from build123d import *

# Parameters (mm, degrees)
SKETCH1_W                       = 39
SKETCH1_H                       = 155
BOSS_EXTRUDE1_DEPTH             = 2
BOSS_EXTRUDE2_DEPTH             = 38
SKETCH3_W                       = 2
SKETCH3_H                       = 2
BOSS_EXTRUDE3_DEPTH             = 38
SKETCH4_W                       = 2
SKETCH4_H                       = 2
BOSS_EXTRUDE4_DEPTH             = 151
SKETCH6_W                       = 35
SKETCH6_H                       = 2.2
CUT_EXTRUDE1_DEPTH              = 160.340045186
SKETCH7_W                       = 35
SKETCH7_H                       = 2.2
CUT_EXTRUDE2_DEPTH              = 89.490112442
SKETCH5_W                       = 31
SKETCH5_H                       = 2
BOSS_EXTRUDE5_DEPTH             = 2
BOSS_EXTRUDE6_REACH             = 91.367
SKETCH8_W                       = 2
SKETCH8_H                       = 2
BOSS_EXTRUDE6_DIRECTION_2_REACH = 91.367
SKETCH10_W                      = 2
SKETCH10_H                      = 2.2
SKETCH10_W_2                    = 2.2
SKETCH10_H_2                    = 2
BOSS_EXTRUDE8_DEPTH             = 2
SKETCH11_W                      = 2
SKETCH11_H                      = 2.2
SKETCH11_W_2                    = 2.2
SKETCH11_H_2                    = 2
BOSS_EXTRUDE9_DEPTH             = 2
FILLET2_R                       = 2.5
SKETCH14_W                      = 36.5
SKETCH14_H                      = 7.75
BOSS_EXTRUDE10_DEPTH            = 2
SKETCH13_W                      = 31
SKETCH13_H                      = 3
CUT_EXTRUDE4_DEPTH              = 2
FILLET3_R                       = 2
FILLET4_R                       = 0.5
SKETCH15_R                      = 5.1
CUT_EXTRUDE5_DEPTH              = 90.367219941
SKETCH16_R                      = 7.1
BOSS_EXTRUDE11_DEPTH            = 1
FILLET5_R                       = 0.5
FILLET7_R                       = 0.5
CUT_EXTRUDE6_DEPTH              = 6
SKETCH18_W                      = 29
SKETCH18_H                      = 3
CUT_EXTRUDE8_DEPTH              = 90.367219986
CUT_EXTRUDE11_DEPTH             = 90.367219986
CUT_EXTRUDE11_DEPTH_BACK        = 90.367219986
SKETCH20_W                      = 5
SKETCH20_H                      = 40
SKETCH21_W                      = 9
SKETCH21_H                      = 31
CUT_EXTRUDE12_DEPTH             = 89.41097217
SKETCH22_W                      = 11
SKETCH22_H                      = 22.8
CUT_EXTRUDE13_DEPTH             = 41.425858061


with BuildPart() as part:
    # Sketch1 → Boss-Extrude1 (new body)
    with BuildSketch(Plane(origin=(0, 0, 0), x_dir=(1, 0, 0), z_dir=(0, 1, 0))):
        Rectangle(SKETCH1_W, SKETCH1_H)
    extrude(amount=BOSS_EXTRUDE1_DEPTH)

    # Sketch2 → Boss-Extrude2 (add)
    with BuildSketch(Plane(origin=(0, 2, 0), x_dir=(1, 0, 0), z_dir=(0, 1, 0))):
        Polygon((-17.5, -77.5), (-17.5, -75.5), (-17.5, 75.5), (17.5, 75.5), (17.5, -75.5), (17.5, -77.5), (19.5, -77.5), (19.5, 77.5), (-19.5, 77.5), (-19.5, -77.5), align=None)
    extrude(amount=BOSS_EXTRUDE2_DEPTH)

    # Sketch3 → Boss-Extrude3 (add)
    with BuildSketch(Plane(origin=(0, 2, 0), x_dir=(1, 0, 0), z_dir=(0, 1, 0))):
        with Locations((-16.5, -76.5)):
            Rectangle(SKETCH3_W, SKETCH3_H)
        with Locations((-16.5, -72.3)):
            Rectangle(SKETCH3_W, SKETCH3_H)
        with Locations((16.5, -76.5)):
            Rectangle(SKETCH3_W, SKETCH3_H)
        with Locations((16.5, -72.3)):
            Rectangle(SKETCH3_W, SKETCH3_H)
    extrude(amount=BOSS_EXTRUDE3_DEPTH)

    # Sketch4 → Boss-Extrude4 (add)
    with BuildSketch(Plane.XY.offset(-75.5)):
        with Locations((-16.5, 39)):
            Rectangle(SKETCH4_W, SKETCH4_H)
        Polygon((-15.5, 33.8), (-17.5, 31.8), (-17.5, 35.8), (-15.5, 35.8), align=None)
        Polygon((15.5, 35.8), (17.5, 35.8), (17.5, 31.8), (15.5, 33.8), align=None)
        with Locations((16.5, 39)):
            Rectangle(SKETCH4_W, SKETCH4_H)
    extrude(amount=BOSS_EXTRUDE4_DEPTH)

    # Sketch6 → Cut-Extrude1 (cut, through all)
    with BuildSketch(Plane.XY.offset(-75.5)):
        with Locations((0, 36.9)):
            Rectangle(SKETCH6_W, SKETCH6_H)
    extrude(amount=CUT_EXTRUDE1_DEPTH, mode=Mode.SUBTRACT)

    # Sketch7 → Cut-Extrude2 (cut, through all)
    with BuildSketch(Plane(origin=(0, 2, 0), x_dir=(1, 0, 0), z_dir=(0, 1, 0))):
        with Locations((0, -74.4)):
            Rectangle(SKETCH7_W, SKETCH7_H)
    extrude(amount=CUT_EXTRUDE2_DEPTH, mode=Mode.SUBTRACT)

    # Sketch5 → Boss-Extrude5 (add)
    with BuildSketch(Plane(origin=(0, 2, 0), x_dir=(1, 0, 0), z_dir=(0, 1, 0))):
        with Locations((0, -76.5)):
            Rectangle(SKETCH5_W, SKETCH5_H)
        with Locations((0, -72.3)):
            Rectangle(SKETCH5_W, SKETCH5_H)
    extrude(amount=BOSS_EXTRUDE5_DEPTH)

    # Boss-Extrude6: up to this face of the body (flat: up to its plane)
    boss_extrude6_end = Plane(part.part.faces().sort_by_distance((17.5, 16.9, -2.1))[0])
    # Sketch8 → Boss-Extrude6 (add, up to the picked face)
    with BuildSketch(Plane(origin=(0, 0, 0), x_dir=(0, 0, -1), z_dir=(1, 0, 0)), mode=Mode.PRIVATE) as boss_extrude6_sk1:
        with Locations((74.5, 39)):
            Rectangle(SKETCH8_W, SKETCH8_H)
    boss_extrude6_tool1 = split(extrude(boss_extrude6_sk1.sketch, amount=BOSS_EXTRUDE6_REACH, mode=Mode.PRIVATE), bisect_by=boss_extrude6_end, keep=Keep.BOTH, mode=Mode.PRIVATE)
    # Sketch8 → Boss-Extrude6 (add, up to the picked face)
    with BuildSketch(Plane(origin=(0, 0, 0), x_dir=(0, 0, -1), z_dir=(1, 0, 0)), mode=Mode.PRIVATE) as boss_extrude6_sk2:
        Polygon((75.5, 35.8), (73.5, 35.8), (73.5, 33.8), (75.5, 31.8), align=None)
    boss_extrude6_tool2 = split(extrude(boss_extrude6_sk2.sketch, amount=BOSS_EXTRUDE6_REACH, mode=Mode.PRIVATE), bisect_by=boss_extrude6_end, keep=Keep.BOTH, mode=Mode.PRIVATE)
    add(boss_extrude6_tool1.solids().sort_by(Axis((0, 39, -74.5), (1, 0, 0)))[0])
    add(boss_extrude6_tool2.solids().sort_by(Axis((0, 34.244444, -74.611111), (1, 0, 0)))[0])

    # Boss-Extrude6 direction 2: up to this face of the body (flat: up to its plane)
    boss_extrude6_direction_2_end = Plane(part.part.faces().sort_by_distance((-17.5, 16.9, -2.1))[0])
    # Sketch8 → Boss-Extrude6 direction 2 (add, up to the picked face)
    with BuildSketch(Plane(origin=(0, 0, 0), x_dir=(0, 0, -1), z_dir=(1, 0, 0)), mode=Mode.PRIVATE) as boss_extrude6_direction_2_sk1:
        with Locations((74.5, 39)):
            Rectangle(SKETCH8_W, SKETCH8_H)
    boss_extrude6_direction_2_tool1 = split(extrude(boss_extrude6_direction_2_sk1.sketch, amount=-BOSS_EXTRUDE6_DIRECTION_2_REACH, mode=Mode.PRIVATE), bisect_by=boss_extrude6_direction_2_end, keep=Keep.BOTH, mode=Mode.PRIVATE)
    # Sketch8 → Boss-Extrude6 direction 2 (add, up to the picked face)
    with BuildSketch(Plane(origin=(0, 0, 0), x_dir=(0, 0, -1), z_dir=(1, 0, 0)), mode=Mode.PRIVATE) as boss_extrude6_direction_2_sk2:
        Polygon((75.5, 35.8), (73.5, 35.8), (73.5, 33.8), (75.5, 31.8), align=None)
    boss_extrude6_direction_2_tool2 = split(extrude(boss_extrude6_direction_2_sk2.sketch, amount=-BOSS_EXTRUDE6_DIRECTION_2_REACH, mode=Mode.PRIVATE), bisect_by=boss_extrude6_direction_2_end, keep=Keep.BOTH, mode=Mode.PRIVATE)
    add(boss_extrude6_direction_2_tool1.solids().sort_by(Axis((0, 39, -74.5), (-1, 0, 0)))[0])
    add(boss_extrude6_direction_2_tool2.solids().sort_by(Axis((0, 34.244444, -74.611111), (-1, 0, 0)))[0])

    # Sketch10 → Boss-Extrude8 (add)
    with BuildSketch(Plane(origin=(-17.5, 0, 0), x_dir=(0, 0, -1), z_dir=(1, 0, 0))):
        with Locations((-76.5, 36.9)):
            Rectangle(SKETCH10_W, SKETCH10_H)
        with Locations((-74.4, 39)):
            Rectangle(SKETCH10_W_2, SKETCH10_H_2)
    extrude(amount=BOSS_EXTRUDE8_DEPTH)

    # Sketch11 → Boss-Extrude9 (add)
    with BuildSketch(Plane.ZY.offset(-17.5)):
        with Locations((76.5, 36.9)):
            Rectangle(SKETCH11_W, SKETCH11_H)
        with Locations((74.4, 39)):
            Rectangle(SKETCH11_W_2, SKETCH11_H_2)
    extrude(amount=BOSS_EXTRUDE9_DEPTH)

    # Fillet2
    fillet2_edges = [part.edges().sort_by_distance(p)[0] for p in [
        (-17.5, 16.9, 71.3),
        (17.5, 16.9, 71.3),
        (19.5, 20, 77.5),
        (-19.5, 20, 77.5),
        (-19.5, 20, -77.5),
        (-17.5, 16.9, -75.5),
        (17.5, 16.9, -75.5),
        (19.5, 20, -77.5),
        (19.5, 40, 0),
        (-19.5, 40, 0),
        (19.5, 0, 0),
        (-19.5, 0, 0),
        (0, 40, -77.5),
        (0, 0, 77.5),
        (0, 0, -77.5),
        (-17.5, 40, 77.5),
        (17.5, 40, 77.5),
    ]]
    fillet(fillet2_edges, radius=FILLET2_R)

    # Sketch14 → Boss-Extrude10 (add)
    with BuildSketch(Plane.XY.offset(-75.5)):
        with Locations((0, 5.125)):
            Rectangle(SKETCH14_W, SKETCH14_H)
    extrude(amount=BOSS_EXTRUDE10_DEPTH)

    # Sketch13 → Cut-Extrude4 (cut)
    with BuildSketch(Plane(origin=(0, 0, -77.5), x_dir=(-1, 0, 0), z_dir=(0, 0, -1))):
        with Locations((0, 5.5)):
            Rectangle(SKETCH13_W, SKETCH13_H)
    extrude(amount=-CUT_EXTRUDE4_DEPTH, mode=Mode.SUBTRACT)

    # Fillet3
    fillet3_edges = [part.edges().sort_by_distance(p)[0] for p in [
        (0, 9, -73.5),
    ]]
    fillet(fillet3_edges, radius=FILLET3_R - 0.0001)  # a hair under: the kernel refuses the full size

    # Fillet4
    fillet4_edges = [part.edges().sort_by_distance(p)[0] for p in [
        (15.5, 5.5, -75.5),
        (15.5, 4, -76.5),
        (0, 7, -75.5),
        (15.5, 7, -76.5),
        (-15.5, 5.5, -75.5),
        (-15.5, 7, -76.5),
        (0, 4, -75.5),
        (-15.5, 4, -76.5),
        (15.5, 5.5, -77.5),
        (0, 4, -77.5),
        (-15.5, 5.5, -77.5),
        (0, 7, -77.5),
    ]]
    fillet(fillet4_edges, radius=FILLET4_R)

    # Sketch15 → Cut-Extrude5 (cut, through all)
    with BuildSketch(Plane.XZ):
        with Locations(Location((0, 38.75, 0), (0, 0, 270))):
            Circle(SKETCH15_R)
        with Locations(Location((0, -38.75, 0), (0, 0, 270))):
            Circle(SKETCH15_R)
    extrude(amount=-CUT_EXTRUDE5_DEPTH, mode=Mode.SUBTRACT)

    # Sketch16 → Boss-Extrude11 (add)
    with BuildSketch(Plane(origin=(0, 2, 0), x_dir=(1, 0, 0), z_dir=(0, 1, 0))):
        with Locations(Location((0, 38.75, 0), (0, 0, 270))):
            Circle(SKETCH16_R)
        with Locations(Location((0, -38.75, 0), (0, 0, 270))):
            Circle(SKETCH16_R)
    extrude(amount=BOSS_EXTRUDE11_DEPTH)

    # Fillet5
    fillet5_edges = [part.edges().sort_by_distance(p)[0] for p in [
        (0, 2, -45.85),
        (0, 3, -45.85),
        (0, 2, 31.65),
        (0, 3, 31.65),
    ]]
    fillet(fillet5_edges, radius=FILLET5_R - 0.0001)  # a hair under: the kernel refuses the full size

    # Fillet7
    fillet7_edges = [part.edges().sort_by_distance(p)[0] for p in [
        (15.5, 40, 0.75),
        (0, 4, 77.5),
        (0, 40, -73.5),
        (-15.5, 40, 0.75),
        (-15.5, 20.75, 77.5),
        (-15.5, 39.267766953, 76.767766953),
        (15.5, 20.75, 77.5),
        (15.5, 39.267766953, 76.767766953),
    ]]
    fillet(fillet7_edges, radius=FILLET7_R)

    # Sketch17 → Cut-Extrude6 (cut)
    with BuildSketch(Plane.XZ):
        Polygon((-17, -77.5), (-17, 70.299999999), (-14.999999999, 71.3), (-14.999999999, 77.5), (14.999999999, 77.5), (14.999999999, 71.3), (17, 70.299999999), (17, -77.5), align=None)
    extrude(amount=-CUT_EXTRUDE6_DEPTH, mode=Mode.SUBTRACT)

    # Sketch18 → Cut-Extrude8 (cut, through all)
    with BuildSketch(Plane.XY):
        with Locations((0, 7.5)):
            Rectangle(SKETCH18_W, SKETCH18_H)
    extrude(amount=-CUT_EXTRUDE8_DEPTH, mode=Mode.SUBTRACT)

    # Sketch20 → Cut-Extrude11 (cut, two sides: drawn at the far end of the back side and taken through both)
    with BuildSketch(Plane.XY.offset(-CUT_EXTRUDE11_DEPTH_BACK)):
        Polygon((19.5, 40), (14.5, 40), (14.5, 6), (14.5, 0), (19.5, 0), align=None)
        with Locations((-17, 20)):
            Rectangle(SKETCH20_W, SKETCH20_H)
    extrude(amount=CUT_EXTRUDE11_DEPTH + CUT_EXTRUDE11_DEPTH_BACK, mode=Mode.SUBTRACT)

    # Sketch21 → Cut-Extrude12 (cut, through all)
    with BuildSketch(Plane.XY):
        with Locations((-10, 24.5)):
            Rectangle(SKETCH21_W, SKETCH21_H)
        with Locations((10, 24.5)):
            Rectangle(SKETCH21_W, SKETCH21_H)
    extrude(amount=-CUT_EXTRUDE12_DEPTH, mode=Mode.SUBTRACT)

    # Sketch22 → Cut-Extrude13 (cut, through all)
    with BuildSketch(Plane.XY.offset(-75.5)):
        with Locations((0, 20.4)):
            Rectangle(SKETCH22_W, SKETCH22_H)
    extrude(amount=-CUT_EXTRUDE13_DEPTH, mode=Mode.SUBTRACT)


solid = part.part
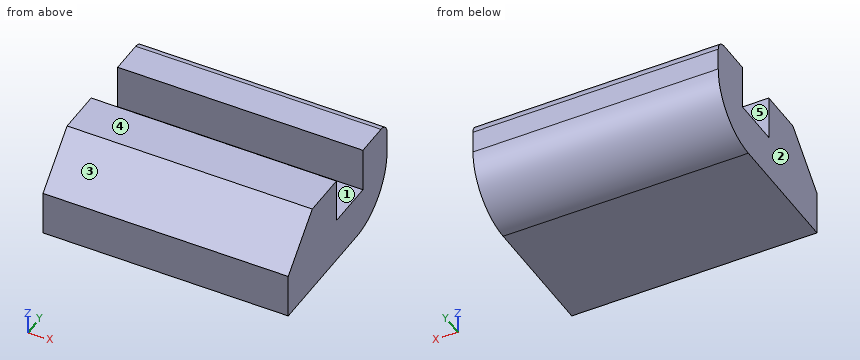
Work out the finished part from the listing and answer in its coordinate system (mm). Face numbers are marked on the shaded views. A direction names the side the tool comes from. Coordinates: 2 decimals unless noted, no trailing zeros. Write each loop counter-clockwise with the first axis right and the second up, starting at its lowest first coordinate (ties: lowest second). Pieces come first, ordered by that corner, then holes. Notation, with made-up numbers: M 58,59 L 109,59 A31 cw 109,97 Z; hole C 1,15.5 d7. An arc over 180 degrees is marked long. Use one line per item in the form item = value. Start each with the question number.
1. A tool of negligible diameter and unlimited length cuts with its end or side. For the marked faces 4 and 5, from which of +Z, -Z, +X, -X, +Y, -Y can it reach the whole face along a straight path? Write none if from no direction.
2. The part is cut by section A-A (z = -74.35). Give the vertices of the cut face in (x, y), plus the area to 4 significant figures.
3. The mould has two halves that part along Y. Classify the marked faces 1, 2 and 3: released by +Y, released by -Y, zero draft, split by the parting line, or undercut.
4. The part is cut by section D-D (z = -76.5). Give the vertices of the cut face in (x, y), plus the area to 3 significant figures.
5. The part is cut by section C-C (y = 33). Give the vertices of the cut face in (x, z), plus the area to 3 significant figures.
6. Each of these flat-tipped pins is pushed along its axis until it touches: P1, Ø1.8, axis at x = 0.5, y = 37, coming from the +Z side; P2, Ø1.6, axis at x = 1.5, z = -74, coming from the -Y side. Where does it stop, or does it pass through?
7. The part is cut by section B-B (x = 5.25). Give the vertices of the cut face in (y, z), plus the area to 3 significant figures.
8. Straight lines are drawn through the part: probe 1 along Z at (x, y) = (-3.25, 37.5); probe 2 along Y at (x, z) = (-2.5, -74.35); probe 3 along Y at (x, z) = (0.25, -76.5). For each, find the intervals that lie inside material, in ascending order. Write a range as from..to.
Evaluation:
q1.face_4 = +Z, +X, -X, +Y, -Y
q1.face_5 = +Z, +X, -X
q2.outline = M -5.5,32.95 L 5.5,32.95 L 5.5,35.8 L -5.5,35.8 Z; M -5.5,38 L 5.5,38 L 5.5,40 L -5.5,40 Z
q2.area = 53.35 mm^2
q3.face_1 = undercut
q3.face_2 = zero draft
q3.face_3 = released by -Y
q4.outline = M -5.5,31.8 L 5.5,31.8 L 5.5,39.5 L -5.5,39.5 Z
q4.area = 84.7 mm^2
q5.outline = M -5.5,-77.5 L 5.5,-77.5 L 5.5,-74.3 L -5.5,-74.3 Z
q5.area = 35.2 mm^2
q6.P1 = -75.5
q6.P2 = 32.5
q7.outline = M 31.8,-77.5 L 37.5,-77.5 A2.5 ccw 40,-75 L 40,-74 A0.5 ccw 39.5,-73.5 L 38,-73.5 L 38,-75.5 L 35.8,-75.5 L 35.8,-73.5 L 33.8,-73.5 L 31.8,-75.5 Z
q7.area = 25.0 mm^2
q8.probe_1 = -77.5..-75.5
q8.probe_2 = 32.95..35.8, 38..40
q8.probe_3 = 31.8..39.5
